from build123d import *

# Parameters (mm, degrees)
BOSS_EXTRUDE2_DEPTH     = 1.000000032
BOSS_EXTRUDE4_DEPTH     = 1.000000032
SKETCH4_R               = 3.175
SKETCH4_R_2             = 0.950000005
CUT_EXTRUDE1_DEPTH      = 1
CUT_EXTRUDE1_DEPTH_BACK = 2.000000032
SKETCH6_W               = 13.430000064
SKETCH6_H               = 9.525
SKETCH6_W_2             = 32.960056
BOSS_EXTRUDE5_DEPTH     = 1.000000032
CUT_EXTRUDE2_DEPTH      = 1
CUT_EXTRUDE2_DEPTH_BACK = 2.000000032


with BuildPart() as part:
    # Sketch2 → Boss-Extrude2 (new body)
    with BuildSketch(Plane(origin=(0, 0, 0), x_dir=(1, 0, 0), z_dir=(0, 1, 0))):
        Polygon((-31.351491175, -35.060458992), (-60.325, 9.840821613), (-60.325, -47.760458992), (0, -47.760458992), (60.325, -47.760458992), (60.325, -2.200955885), (-26.791523135, -35.060458992), align=None)
    extrude(amount=BOSS_EXTRUDE2_DEPTH)

    # Sketch5 → Boss-Extrude4 (add)
    with BuildSketch(Plane(origin=(0, 0, 0), x_dir=(1, 0, 0), z_dir=(0, 1, 0))):
        with BuildLine():
            Line((60.325, -47.760458992), (75.025000064, -47.760458992))
            Line((75.025000064, -47.760458992), (107.985056064, -47.760458992))
            ThreePointArc((107.985056064, -47.760458992), (120.685056064, -35.060458992), (107.985056064, -22.360458992))
            Line((107.985056064, -22.360458992), (75.025000064, -22.360458992))
            Line((75.025000064, -22.360458992), (75.025000064, -35.060458992))
            Line((75.025000064, -35.060458992), (60.325, -35.060458992))
            Line((60.325, -35.060458992), (60.325, -47.760458992))
        make_face()
    extrude(amount=BOSS_EXTRUDE4_DEPTH)

    # Sketch4 → Cut-Extrude1 (cut, two sides)
    with BuildSketch(Plane(origin=(0, 1.000000032, 0), x_dir=(1, 0, 0), z_dir=(0, 1, 0))) as cut_extrude1_sk:
        with Locations((107.985056064, -35.060458992)):
            Circle(SKETCH4_R)
        with Locations((107.985056064, -42.060458962)):
            Circle(SKETCH4_R_2)
        with Locations((107.985056064, -28.060459022)):
            Circle(SKETCH4_R_2)
        with Locations((100.985056094, -35.060458992)):
            Circle(SKETCH4_R_2)
        with Locations((114.985056034, -35.060458992)):
            Circle(SKETCH4_R_2)
    extrude(amount=CUT_EXTRUDE1_DEPTH, mode=Mode.SUBTRACT)
    extrude(cut_extrude1_sk.sketch, amount=-CUT_EXTRUDE1_DEPTH_BACK, mode=Mode.SUBTRACT)

    # Sketch6 → Boss-Extrude5 (add)
    with BuildSketch(Plane(origin=(0, 1.000000032, 0), x_dir=(1, 0, 0), z_dir=(0, 1, 0))):
        with Locations((67.040000032, -52.522958992)):
            Rectangle(SKETCH6_W, SKETCH6_H)
        with Locations((91.505028064, -17.597958992)):
            Rectangle(SKETCH6_W_2, SKETCH6_H)
    extrude(amount=-BOSS_EXTRUDE5_DEPTH)

    # Sketch8 → Cut-Extrude2 (cut, two sides)
    with BuildSketch(Plane(origin=(0, 1.000000032, 0), x_dir=(1, 0, 0), z_dir=(0, 1, 0))) as cut_extrude2_sk:
        Polygon((-26.791523135, -35.060458992), (2.18198569, -24.131933967), (2.18198569, -35.060458992), align=None)
    extrude(amount=CUT_EXTRUDE2_DEPTH, mode=Mode.SUBTRACT)
    extrude(cut_extrude2_sk.sketch, amount=-CUT_EXTRUDE2_DEPTH_BACK, mode=Mode.SUBTRACT)


solid = part.part
Geometry check sheet. Reference: the model listing, model coordinates, mm. A direction names the side the tool comes from. Give positions to 0.01 mm unless a question says otherwise; leave off trailing zeros. Order: outer loops, then holes, each group sorted by start corner. A loop starts at its lowest first (then second) coordinate and runs counter-clockwise, first axis right, second up. Notation, with made-up numbers: (57, 80.25) - (112, 80.25) arc R12 ccw to (112, 93.25) - close; hole circle Ø9 at (32.5, 85). An arc over 180 degrees is marked (long way). Answer as a JSON object with one key per item and string values.
(1) Draft check along X on faces 1 (the flat face through (29, 1, 31)), 2 (the cylindrical face through (104.813, 0.507, 34.921)), 3 (the cylindrical face through (120.68, 0.49, 35.34)). Enter one of: released by +X, released by -X, zero draft, split by the parting line, or undercut.
Report:
{"face 1": "zero draft", "face 2": "undercut", "face 3": "released by +X"}
(2) Cross-section at D-D (z = -5). Record the cut outline in (x, y) (3 decimals), then the cut area to 3 significant figures.
Report:
{"outline": "(-60.325, 0) - (-57.201, 0) - (-57.201, 1) - (-60.325, 1) - close", "area": "3.12 mm^2"}
(3) Cross-section at B-B (y = 0.4). State how many separate pieces and enclosed holes the cut face has, then the cut area to 3 significant figures.
Report:
{"separate pieces": "1", "enclosed holes": "5", "area": "5,130 mm^2"}
(4) Material ranges on line 1 (Z direction, x = 70.5, y = 0.5); line 2 (Z direction, x = 110.5, y = 0.3); line 3 (X direction, y = 0.75, z = 31) (3 decimals), recorded low to high.
Report:
{"line 1": "35.06 to 57.29", "line 2": "22.61 to 33.12, 37 to 47.51", "line 3": "-60.325 to -33.972, 2.182 to 60.325, 75.025 to 120.018"}
(5) Cross-section at C-C (x = 82.5). Record the cut outline in (y, z).
Report:
{"outline": "(0, 12.84) - (1, 12.84) - (1, 47.76) - (0, 47.76) - close"}
(6) Cross-section at A-A (z = 8.5). Record the cut outline in (x, y) (3 decimals), then the cut area to 3 significant figures.
Report:
{"outline": "(-60.325, 0) - (-48.49, 0) - (-48.49, 1) - (-60.325, 1) - close; (43.625, 0) - (60.325, 0) - (60.325, 1) - (43.625, 1) - close", "area": "28.5 mm^2"}
(7) Depth check by flat-ended pin: pin 1 Ø1.7 at (x, z) = (107.99, 42.06) entering from -Y; pin 2 Ø0.5 at (x, y) = (20.5, 0.5) entering from +Z; pin 3 Ø0.5 at (y, z) = (0.5, 50.5) entering from -X (3 decimals); pin 4 Ø2.5 at (x, z) = (100.99, 35.06) entering from -Y. Enter the tip coordinate at first touch or a pass-through.
Report:
{"pin 1": "through", "pin 2": "z = 47.76", "pin 3": "x = 60.325", "pin 4": "y = 0"}
(8) Tool access check on faces 4 (the flat face through (-45.64, 0.49, 12.92)), 5 (the flat face through (29, 0, 31)). Record the directions out of +Z, -Z, +X, -X, +Y, -Y that give a thin tool (end or side, any length) a straight path to the whole face; none if there is none.
Report:
{"face 4": "-Z, +Y, -Y", "face 5": "+Z, -Z, +X, -X, -Y"}
